Design review of the part built by this model. Coordinates are the model's own, in mm. A direction names the side the tool comes from. Coordinates: 2 decimals unless noted, no trailing zeros. Write each loop counter-clockwise with the first axis right and the second up, starting at its lowest first coordinate (ties: lowest second). Pieces come first, ordered by that corner, then holes. Notation, with made-up numbers: (13.25, 7) - (30.25, 7) arc R19 cw to (30.25, 39) - close; hole circle Ø2 at (46, -14.75). An arc over 180 degrees is marked (long way). One line per item, written item: value.
Autodesk Inventor part; units mm, degrees
ref_plane "YZ Plane" through (0, 0, 0) normal (1, 0, 0) x (0, 1, 0)
ref_plane "XZ Plane" through (0, 0, 0) normal (0, 1, 0) x (-1, 0, 0)
ref_plane "XY Plane" through (0, 0, 0) normal (0, 0, 1) x (1, 0, 0)
sketch "Sketch1" plane through (0, 0, 0) normal (0, 0, 1) x (1, 0, 0)
  circle A0 centre (0, 0) radius 5
  dimension "d0" = 10
extrude "Extrusion1" add sketch "Sketch1" along normal blind 6
sketch "Sketch2" plane through (0, 0, 6) normal (0, 0, 1) x (1, 0, 0)
  circle A0 centre (0, 0) radius 5
  circle A1 centre (0, 0) radius 3
  dimension "d3" = 6
extrude "Extrusion2" add sketch "Sketch2" along normal blind 25 contours A1
thread "Thread1"
chamfer "Chamfer1" distance 1 angle 45 1 edges at (-3, 0, 31)
chamfer "Chamfer2" distance 0.2 angle 45 1 edges at (-5, 0, 6)
fillet "Fillet1" radius 1 1 edges at (-5, 0, 0)
sketch "Sketch3" plane through (0, 0, 0) normal (0, 0, -1) x (-1, 0, 0)
  circle A0 centre (0, 0) radius 4
  line L0 (1.5588, 2.4297) -> (2.8836, -0.135)
  line L1 (2.8836, -0.135) -> (1.3248, -2.5648)
  line L2 (1.3248, -2.5648) -> (-1.5588, -2.4297)
  line L3 (-1.5588, -2.4297) -> (-2.8836, 0.135)
  line L4 (-2.8836, 0.135) -> (-1.3248, 2.5648)
  line L5 (-1.3248, 2.5648) -> (1.5588, 2.4297)
  dimension "d15" = 5
extrude "Extrusion3" cut sketch "Sketch3" against normal blind 5 contours L0 L1 L2 L3 L4 L5
properties part number "PERNO PARKER M6"
1. Mouldability with a two-part tool opening along Y and no side actions: class faces 4 (the face through (-2.21, 1.17, 2.46)), 5 (the face through (0, 0, 31)), 6 (the face through (-3, 0, 18)) as released by +Y, released by -Y, zero draft, split by the parting line, or undercut.
Answer block:
face 4: undercut
face 5: zero draft
face 6: split by the parting line
2. Consider section B-B, the plane x = 0. Write out the cut boundary in (y, z), then the cut area to 3 significant figures.
Answer block:
outline: (-5, 1) arc R1 ccw to (-4, 0) - (-2.5, 0) - (-2.5, 5) - (2.5, 5) - (2.5, 0) - (4, 0) arc R1 ccw to (5, 1) - (5, 5.8) - (4.8, 6) - (3, 6) - (3, 30) - (2, 31) - (-2, 31) - (-3, 30) - (-3, 6) - (-4.8, 6) - (-5, 5.8) - close
area: 184 mm^2
3. Consider section A-A, the plane z = 3. Write out the cut boundary in (x, y) (3 decimals).
Answer block:
outline: circle Ø10 at (0, 0); hole (-2.884, -0.135) - (-1.325, -2.565) - (1.559, -2.43) - (2.884, 0.135) - (1.325, 2.565) - (-1.559, 2.43) - close
4. Insertion check: pin 1 Ø3 at (x, z) = (-1.5, 12) entering from +Y; pin 2 Ø1.5 at (y, z) = (3, 25) entering from -X; pin 3 Ø1.5 at (x, y) = (3.5, 3.5) entering from +Z. Each pin has a flat end and moves straight along its axis. Give the tip position at first contact, or say it passes through.
Answer block:
pin 1: stops at y = 3
pin 2: stops at x = -1.98
pin 3: stops at z = 6
5. Wall thickness on line 1 along Z through (x, y) = (1.25, 1); line 2 along Y through (x, z) = (3, 5); line 3 along Z through (x, y) = (-3.75, -1): over which ranges is each line inside the solid? List them lowest first.
Answer block:
line 1: z = 5 to 31
line 2: y = -4 to 4
line 3: z = 0 to 6
6. For faces 1 (the face through (0, -3, 0)), 2 (the face through (1, -3, 6)), 3 (the face through (-2.115, -1.333, 2.465)), list the 3-axis set-ups (+Z, -Z, +X, -X, +Y, -Y) from which the entire face can be reached by the end or side of a thin tool; tool diameter is ignored.
Answer block:
face 1: -Z, +X, -X, +Y, -Y
face 2: +Z
face 3: -Z
7. Consider section C-C, the plane z = 19.5. Write out the cut boundary in (x, y).
Answer block:
outline: circle Ø6 at (0, 0)
